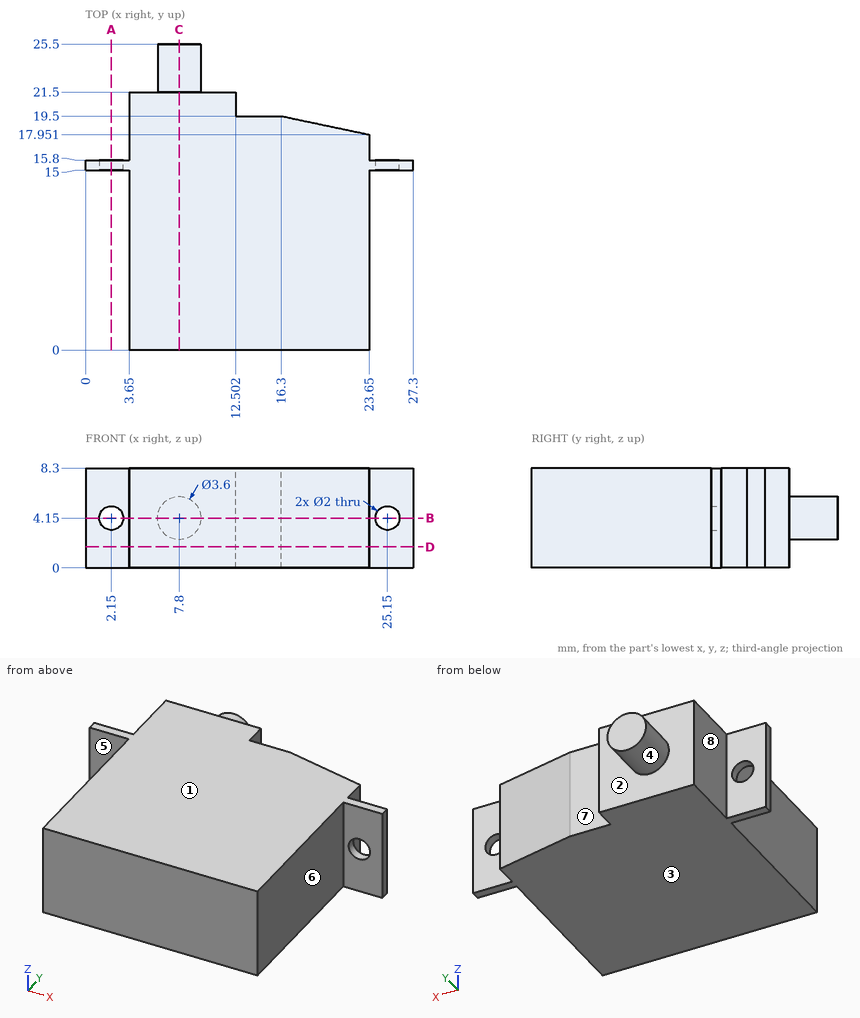
Check sheet for the drawn part. Datum: minimum x, y, z corner. Units: mm. A direction names the side the tool comes from. Give positions to 0.01 mm unless a question says otherwise; leave off trailing zeros. Write each loop counter-clockwise with the first axis right and the second up, starting at its lowest first coordinate (ties: lowest second). Pieces come first, ordered by that corner, then holes. Notation, with made-up numbers: M -13.75,-2.75 L 25.25,-2.75 A7 cw 25.25,3.25 Z; hole C 81,85.25 d9. An arc over 180 degrees is marked long. One line per question, with ' | ' between items.
1. Mould release check, pull along Z, two halves, no side actions. Record for the marked faces 1, 2 and 3: released by +Z, released by -Z, zero draft, split by the parting line, or undercut.
Ans:
face 1: released by +Z | face 2: zero draft | face 3: released by -Z
2. Gauge pin test, flat ends, axial feed: pin 1 (2 mm diameter, centred on x = 20.5, z = 1.5, fed in from +Y) (1 decimal); pin 2 (4 mm diameter, centred on x = 1.5, z = 3, fed in from +Y); pin 3 (4 mm diameter, centred on x = 15, z = 4, fed in from +Y); pin 4 (2 mm diameter, centred on y = 16.5, z = 1, fed in from -X). Record the tip position at first contact, or that the pin passes through.
Ans:
pin 1: y = 18.8 | pin 2: y = 15.8 | pin 3: y = 19.5 | pin 4: x = 0
3. Set-up check for the marked faces 4, 5, 6, 7 and 8: record each of +Z, -Z, +X, -X, +Y, -Y from which the full face is reachable in a straight line by a thin tool's end or side.
Ans:
face 4: +Y | face 5: +Z, -Z, -X, -Y | face 6: +Z, -Z, +X, -Y | face 7: +Z, -Z, +X, +Y | face 8: +Z, -Z, -X, +Y
4. Cross-section at B-B (z = 4.15). Enter the section's corners in (x, y).
Ans:
outline: M 0,15 L 1.15,15 L 1.15,15.8 L 0,15.8 Z; M 3.15,15 L 3.65,15 L 3.65,0 L 23.65,0 L 23.65,15 L 24.15,15 L 24.15,15.8 L 23.65,15.8 L 23.65,17.95 L 16.3,19.5 L 12.5,19.5 L 12.5,21.5 L 9.6,21.5 L 9.6,25.5 L 6,25.5 L 6,21.5 L 3.65,21.5 L 3.65,15.8 L 3.15,15.8 Z; M 26.15,15 L 27.3,15 L 27.3,15.8 L 26.15,15.8 Z
5. Cross-section at D-D (z = 1.75). Enter the section's corners in (x, y).
Ans:
outline: M 0,15 L 3.65,15 L 3.65,0 L 23.65,0 L 23.65,15 L 27.3,15 L 27.3,15.8 L 23.65,15.8 L 23.65,17.95 L 16.3,19.5 L 12.5,19.5 L 12.5,21.5 L 3.65,21.5 L 3.65,15.8 L 0,15.8 Z
6. Cross-section at C-C (x = 7.8). Enter the section's corners in (y, z).
Ans:
outline: M 0,0 L 21.5,0 L 21.5,2.35 L 25.5,2.35 L 25.5,5.95 L 21.5,5.95 L 21.5,8.3 L 0,8.3 Z
7. Scan lines: line 1 along Z through (x, y) = (2.15, 15.65); line 2 along X through (y, z) = (20.5, 3.5); line 3 along Y through (x, z) = (14.25, 7). Record each from-to range of solid material in increasing order. Write a range as from..to.
Ans:
line 1: 0..3.15, 5.15..8.3 | line 2: 3.65..12.5 | line 3: 0..19.5
8. Cross-section at A-A (x = 2.15). Enter the section's corners in (y, z).
Ans:
outline: M 15,0 L 15.8,0 L 15.8,3.15 L 15,3.15 Z; M 15,5.15 L 15.8,5.15 L 15.8,8.3 L 15,8.3 Z
